from build123d import *

# Parameters (mm, degrees)
F0_W     = 152.4
F0_H     = 76.2
F1_DEPTH = 19.05
F2_R     = 6.35
F3_DEPTH = 19.05
F4_SIZE  = 3.81
F7_R     = 25.4
F8_DEPTH = 25.4
F9_R     = 5.07999


# Not quite as in the source:
# - a fillet or chamfer is up to 0.001 mm smaller than in the source, because OpenCascade refuses the exact size


with BuildPart() as f1:
    # F0 (on Top) → F1 (new body)
    with BuildSketch(Plane.XY):
        Rectangle(F0_W, F0_H)
    extrude(amount=F1_DEPTH)

    # F2 (on face) → F3 (cut, through all)
    with BuildSketch(Plane.XY.offset(19.05)):
        with Locations((-60.96, 22.86)):
            Circle(F2_R)
        with Locations((-60.96, -22.86)):
            Circle(F2_R)
        with Locations((60.96, 22.86)):
            Circle(F2_R)
        with Locations((60.96, -22.86)):
            Circle(F2_R)
    extrude(amount=-F3_DEPTH, mode=Mode.SUBTRACT)

    # F4
    f4_edges = [f1.edges().sort_by_distance(p)[0] for p in [
        (0, -38.1, 19.05),
        (76.2, 0, 19.05),
        (0, 38.1, 19.05),
        (-76.2, 0, 19.05),
    ]]
    chamfer(f4_edges, length=F4_SIZE)

    # F5 (on Front) → F6 (revolve)
    with BuildSketch(Plane.XZ):
        Polygon((0, 69.85), (0, 19.05), (25.4, 19.05), (25.4, 44.45), (20.32, 44.45), (20.32, 69.85), align=None)
    revolve(axis=Axis((0, 0, 44.45), (0, 0, 1)))

    # F7 (on face) → F8 (join)
    with BuildSketch(Plane.XY.offset(69.85)):
        Circle(F7_R)
    extrude(amount=F8_DEPTH)

    # F9 (radius 5.08 in the source; OpenCascade refuses exactly that, so slightly less here)
    f9_edges = [f1.edges().sort_by_distance(p)[0] for p in [
        (-25.4, 0, 19.05),
        (-20.32, 0, 44.45),
        (-20.32, 0, 69.85),
    ]]
    fillet(f9_edges, radius=F9_R)


solid = f1.part
CAD build for the part. Positions are in the model's coordinates, mm. A direction names the side the tool comes from. Round coordinates to 2 decimals unless told otherwise and drop trailing zeros. Write each loop counter-clockwise with the first axis right and the second up, starting at its lowest first coordinate (ties: lowest second). Pieces come first, ordered by that corner, then holes. Notation, with made-up numbers: M -21,-4 L 4,-4 A28 ccw 4,28 Z; hole C 67,-34 d5. An arc over 180 degrees is marked long. Use a Markdown table: item, result. Add a question column.
1. Pull direction Z, two halves, no side cores. Call faces 3 (the face through (-2.645, 20.147, 57.257)), 4 (the face through (74.32, -0.53, 17.12)), 5 (the face through (76.2, -1, 8)): released by +Z, released by -Z, zero draft, split by the parting line, or undercut.
2. Slice it at A-A on x = -60.96. Give the cut face in (y, z), then the cut area to 3 significant figures.
3. Drill centre lines: probe 1 along Y at (x, z) = (60.96, 9.5); probe 2 along Y at (x, z) = (60, 5); probe 3 along Z at (x, y) = (33, 33). Where is each one in solid material? Low to high.
4. Flat gauge pins, fed straight in: P1, Ø11.5, axis at x = -60.96, y = 22.86, coming from the -Z side; P2, Ø1.5, axis at y = -1, z = 85, coming from the +X side; P3, Ø2, axis at y = -2, z = 20, coming from the -X side; P4, Ø12, axis at y = 21, z = 41, coming from the -X side. Where does each tip first touch, or does it go through?
5. 3-axis set-ups, long thin cutter, end or side, ignore diameter. For faces 1 (the face through (-1, -38.1, 8)), 2 (the face through (-5.506, -24.796, 82.372)): which of +Z, -Z, +X, -X, +Y, -Y reach the whole face in a straight line?
6. Slice it at D-D on x = 59. Give the cut face in (y, z).
Reply:
| question | item | result |
|---|---|---|
| 1 | face 3 | undercut |
| 1 | face 4 | released by +Z |
| 1 | face 5 | zero draft |
| 2 | outline | M -38.1,0 L -29.21,0 L -29.21,19.05 L -34.29,19.05 L -38.1,15.24 Z; M -16.51,0 L 16.51,0 L 16.51,19.05 L -16.51,19.05 Z; M 29.21,0 L 38.1,0 L 38.1,15.24 L 34.29,19.05 L 29.21,19.05 Z |
| 2 | area | 953 mm^2 |
| 3 | probe 1 | y = -38.1 to -29.21, -16.51 to 16.51, 29.21 to 38.1 |
| 3 | probe 2 | y = -38.1 to -29.14, -16.58 to 16.58, 29.14 to 38.1 |
| 3 | probe 3 | z = 0 to 19.05 |
| 4 | P1 | passes through |
| 4 | P2 | stops at x = 25.4 |
| 4 | P3 | stops at x = -72.44 |
| 4 | P4 | stops at x = -20.5 |
| 5 | face 1 | +Z, -Z, +X, -X, -Y |
| 5 | face 2 | +Z |
| 6 | outline | M -38.1,0 L -28.9,0 L -28.9,19.05 L -34.29,19.05 L -38.1,15.24 Z; M -16.82,0 L 16.82,0 L 16.82,19.05 L -16.82,19.05 Z; M 28.9,0 L 38.1,0 L 38.1,15.24 L 34.29,19.05 L 28.9,19.05 Z |
